For this review, use the dimensioned drawing (mm, ordinates from the lowest corner) and the shaded views. A direction names the side the tool comes from. Give positions to 0.01 mm unless a question says otherwise; leave off trailing zeros. Loops run counter-clockwise (first coordinate to the right, second up) from the corner with the lowest first, then second, coordinate; pieces in that order, holes last. Notation, with made-up numbers: M 29.25,11 L 33.25,11 A13 ccw 33.25,28 Z; hole C 27,31.5 d6. An arc over 180 degrees is marked long. Use CSV: the item, a comma, the result in double quotes. Start each with the question number.
1. Take a section at A-A, the plane z = 35. Write out the cut boundary in (x, y).
2. The part is to be moulded in two halves that separate along Z. For the marked faces 1, 2 and 3, say which applies: pulls with the +Z half, pulls with the -Z half, needs draft (parallel to the pull), parting line crosses it, or undercut.
3. Take a section at C-C, the plane z = 65. Write out the cut boundary in (x, y).
4. Take a section at D-D, the plane y = 6.5. Write out the cut boundary in (x, z), and give its area (3 significant figures).
5. Insertion check: P1, Ø1, axis at x = 17, y = 26, coming from the -Z side; P2, Ø9, axis at x = 35, z = 5, coming from the -Y side; P3, Ø4, axis at x = 14.5, y = 15, coming from the +Z side; P4, Ø1, axis at y = 12.5, z = 14, coming from the +X side. Each pin has a flat end and moves straight along its axis. Give the tip position at first contact, or say it passes through.
6. Tool access review of the marked faces 4 and 5: name each direction out of +Z, -Z, +X, -X, +Y, -Y from which nothing blocks a thin tool from reaching the whole face with its end or side.
7. To check wall thickness, follow line 1 (X direction, y = 3.5, z = 35); line 2 (Y direction, x = 9, z = 20.5); line 3 (X direction, y = 9, z = 41). State the ranges of each line that lie inside material, in increasing order. Write a range as [from, to].
8. Take a section at B-B, the plane x = 35. Write out the cut boundary in (y, z).
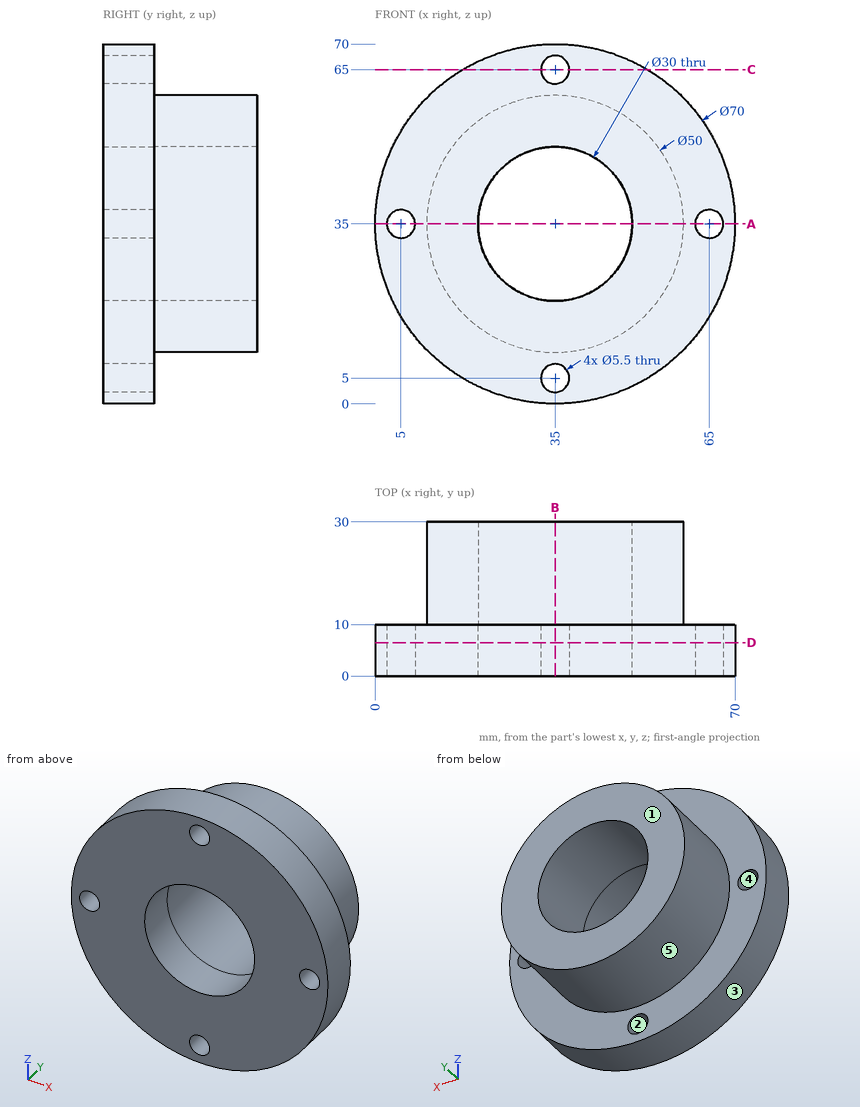
Result set:
1,outline,"M 0,0 L 2.25,0 L 2.25,10 L 0,10 Z; M 7.75,0 L 20,0 L 20,30 L 10,30 L 10,10 L 7.75,10 Z; M 50,0 L 62.25,0 L 62.25,10 L 60,10 L 60,30 L 50,30 Z; M 67.75,0 L 70,0 L 70,10 L 67.75,10 Z"
2,face 1,"needs draft"
2,face 2,"undercut"
2,face 3,"parting line crosses it"
3,outline,"M 16.97,0 L 32.25,0 L 32.25,10 L 16.97,10 Z; M 37.75,0 L 53.03,0 L 53.03,10 L 37.75,10 Z"
4,outline,"C 35,35 d70; hole C 5,35 d5.5; hole C 35,35 d30; hole C 35,5 d5.5; hole C 35,65 d5.5; hole C 65,35 d5.5"
4,area,"3,050 mm2"
5,P1,"z = 17.15"
5,P2,"y = 0"
5,P3,"z = 51.82"
5,P4,"x = 49.31"
6,face 4,"+Y, -Y"
6,face 5,"+Y"
7,line 1,"[0, 2.25], [7.75, 20], [50, 62.25], [67.75, 70]"
7,line 2,"[0, 10]"
7,line 3,"[0.52, 21.25], [48.75, 69.48]"
8,outline,"M 0,0 L 10,0 L 10,2.25 L 0,2.25 Z; M 0,7.75 L 10,7.75 L 10,10 L 30,10 L 30,20 L 0,20 Z; M 0,50 L 30,50 L 30,60 L 10,60 L 10,62.25 L 0,62.25 Z; M 0,67.75 L 10,67.75 L 10,70 L 0,70 Z"
